Autodesk Inventor part; units mm, degrees
ref_plane "YZ Plane" through (0, 0, 0) normal (1, 0, 0) x (0, 1, 0)
ref_plane "XZ Plane" through (0, 0, 0) normal (0, 1, 0) x (-1, 0, 0)
ref_plane "XY Plane" through (0, 0, 0) normal (0, 0, 1) x (1, 0, 0)
sketch "Sketch1" plane through (0, 0, 0) normal (1, 0, 0) x (0, 1, 0)
  line L0 (0, 0) -> (-4, 0)
  line L1 (-4, 0) -> (-4, -50)
  line L2 (-4, -50) -> (0, -50)
  line L3 (0, -50) -> (0, 0)
  line L4 (0, 0) -> (-7, 0)
  line L5 (-7, 0) -> (-7, 4.4)
  line L6 (-7, 4.4) -> (0, 4.4)
  line L7 (0, 4.4) -> (0, 0)
  circle A0 centre (0, 0) radius 7
  point P0 (-5.4443, 4.4)
  dimension "d0" = 4
  dimension "d1" = 50
  dimension "d2" = 7
  dimension "d3" = 4.4
revolve "Revolution1" add sketch "Sketch1" angle 360 about axis through (0, 0, 4.4) along (0, 0, -1) contours L3 A0 L1 L0 | L0 L4 A0 L6 L7 | L3 L2 L1 A0
sketch "Sketch2" plane through (0, 0, 4.4) normal (0, 0, 1) x (1, 0, 0)
  line L0 (2.5, -1.4434) -> (0, -2.8868)
  line L1 (0, -2.8868) -> (-2.5, -1.4434)
  line L2 (-2.5, -1.4434) -> (-2.5, 1.4434)
  line L3 (-2.5, 1.4434) -> (0, 2.8868)
  line L4 (0, 2.8868) -> (2.5, 1.4434)
  line L5 (2.5, 1.4434) -> (2.5, -1.4434)
  point P0 (0, 0)
  point P1 (0, 0)
  dimension "d5" = 5
extrude "Extrusion1" cut sketch "Sketch2" against normal blind 2.6
thread "Thread1"
properties part number "M8 x 50 Button Head Bolt"
Read the model definition and answer for the solid it produces. Units are mm, in the model's axes. A direction names the side the tool comes from. Coordinates: 2 decimals unless noted, no trailing zeros. Loops run counter-clockwise (first coordinate to the right, second up) from the corner with the lowest first, then second, coordinate; pieces in that order, holes last. Notation, with made-up numbers: (46.5, -24) -> (84.5, -24) arc R5 cw to (84.5, -19) -> close; hole circle Ø2 at (20.25, 62.5). An arc over 180 degrees is marked (long way). Write item = value, one per line. Start each with the question number.
1) The part is cut by section D-D, the plane y = 4.5. Determine the outline of the cut face in (x, z), plus the area to 3 significant figures.
2) The part is cut by section B-B, the plane x = -1.25. Determine the outline of the cut face in (y, z).
3) Given P1, Ø2, axis at x = 1.5, z = -1.5, coming from the -Y side; P2, Ø3, axis at y = 0, z = 3, coming from the -X side; P3, Ø1.5, axis at y = -3, z = -29, coming from the -X side, each flat-ended and moving along its own axis, determine where each tip first touches the part or whether it passes through.
4) The part is cut by section C-C, the plane z = -32. Determine the outline of the cut face in (x, y).
5) The part is cut by section A-A, the plane y = 0. Determine the outline of the cut face in (x, z).
6) Find the intervals of material crossed by L1, parallel to Z at x = -4.5, y = 0.75; L2, parallel to Z at x = 0, y = -1; L3, parallel to Y at x = 0, z = -26, in increasing order. Write a range as from..to.
7) For faces 1 (the face through (3, -3, 0)), 2 (the face through (-1.29, -2.34, 4.4)), 3 (the face through (1.233, 2.175, 3.118)), determine the directions among +Z, -Z, +X, -X, +Y, -Y from which every point of the face is accessible in a straight line to the end or side of a thin tool.
8) The mould has two halves that part along X. Classify faces 4 (the face through (0, 0, -50)), 5 (the face through (3.905, 0.867, -25.35)), 6 (the face through (1.267, -2.155, 3.118)): pulls with the +X half, pulls with the -X half, needs draft (parallel to the pull), parting line crosses it, or undercut.
Result:
q1.outline = (-5.36, 0) -> (5.36, 0) arc R5.36 ccw to (3.06, 4.4) -> (-3.06, 4.4) arc R5.36 ccw to start
q1.area = 41.2 mm²
q2.outline = (-6.89, 0) -> (-3.8, 0) -> (-3.8, -50) -> (3.8, -50) -> (3.8, 0) -> (6.89, 0) arc R6.89 ccw to (5.3, 4.4) -> (2.17, 4.4) -> (2.17, 1.8) -> (-2.17, 1.8) -> (-2.17, 4.4) -> (-5.3, 4.4) arc R6.89 ccw to start
q3.P1 = -3.97
q3.P2 = -6.84
q3.P3 = -3.31
q4.outline = circle Ø8 at (0, 0)
q5.outline = (-7, 0) -> (-4, 0) -> (-4, -50) -> (4, -50) -> (4, 0) -> (7, 0) arc R7 ccw to (5.44, 4.4) -> (2.5, 4.4) -> (2.5, 1.8) -> (-2.5, 1.8) -> (-2.5, 4.4) -> (-5.44, 4.4) arc R7 ccw to start
q6.L1 = 0..4.4
q6.L2 = -50..1.8
q6.L3 = -4..4
q7.face_1 = -Z
q7.face_2 = +Z, +X, -X, +Y, -Y
q7.face_3 = +Z
q8.face_4 = needs draft
q8.face_5 = parting line crosses it
q8.face_6 = undercut
